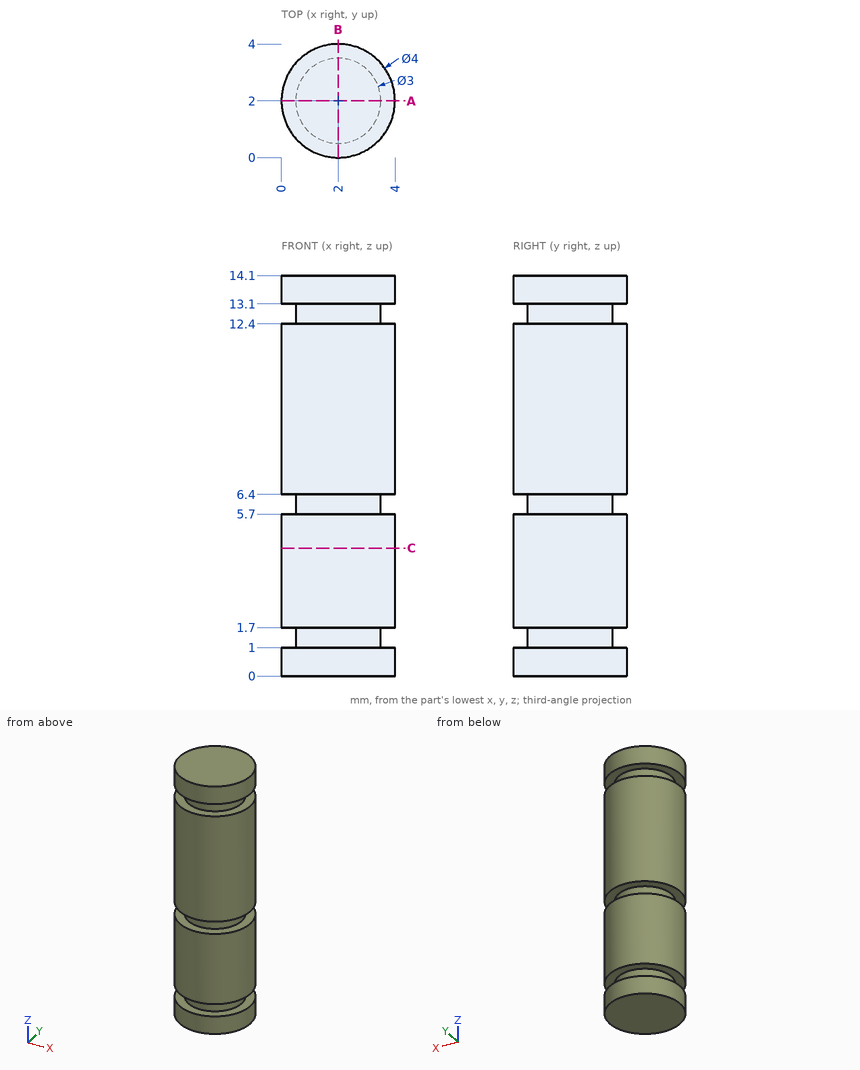
Answer from the drawing. Dimensions are ordinates in mm from the lowest x, y and z of the part. Coordinates: 2 decimals unless noted, no trailing zeros. Loops run counter-clockwise (first coordinate to the right, second up) from the corner with the lowest first, then second, coordinate; pieces in that order, holes last.
1) Section C-C (z = 4.5) is taken. Give the vertices of the cut face in (x, y).
Results:
outline: circle Ø4 at (2, 2)
2) Section A-A (y = 2) is taken. Give the vertices of the cut face in (x, z), plus the area to 3 significant figures.
Results:
outline: (0, 0) - (4, 0) - (4, 1) - (3.5, 1) - (3.5, 1.7) - (4, 1.7) - (4, 5.7) - (3.5, 5.7) - (3.5, 6.4) - (4, 6.4) - (4, 12.4) - (3.5, 12.4) - (3.5, 13.1) - (4, 13.1) - (4, 14.1) - (0, 14.1) - (0, 13.1) - (0.5, 13.1) - (0.5, 12.4) - (0, 12.4) - (0, 6.4) - (0.5, 6.4) - (0.5, 5.7) - (0, 5.7) - (0, 1.7) - (0.5, 1.7) - (0.5, 1) - (0, 1) - close
area: 54.3 mm2
3) Consider probe 1 along Z at (x, y) = (2.55, 0.45); probe 2 along X at (y, z) = (1.9, 10.25); probe 3 along X at (y, z) = (2.9, 7.25). Determine where each line is inside the solid, lowest interval first.
Results:
probe 1: z = 0 to 1, 1.7 to 5.7, 6.4 to 12.4, 13.1 to 14.1
probe 2: x = 0 to 4
probe 3: x = 0.21 to 3.79
